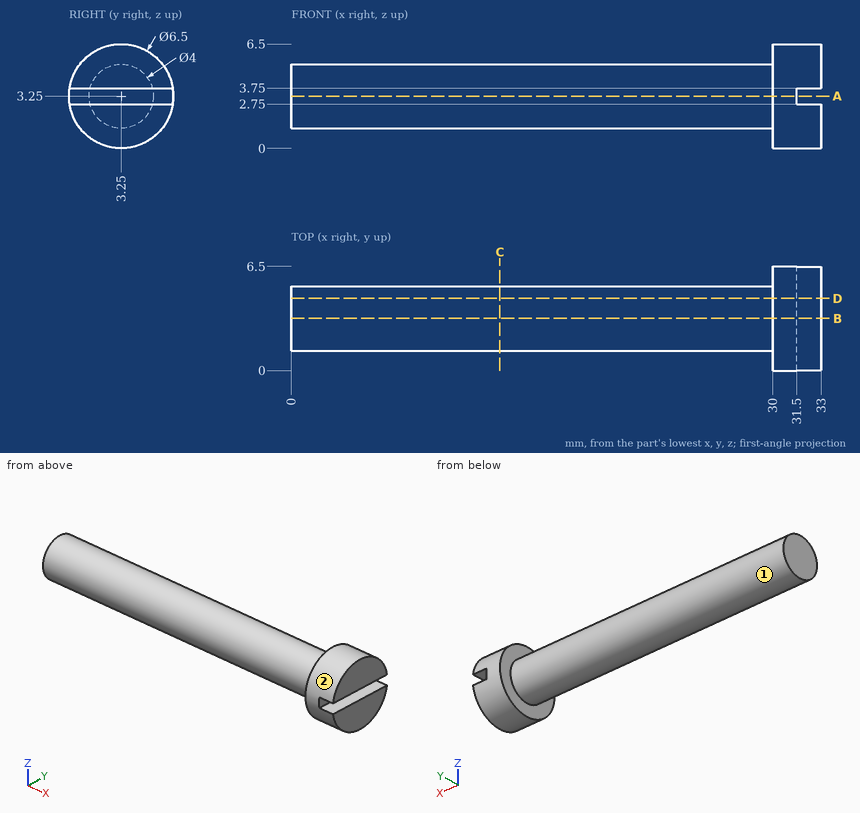
Source: three-view drawing plus pictorial views. Frame: mm from the lowest corner of the part. A direction names the side the tool comes from. Give positions to 0.01 mm unless a question says otherwise; leave off trailing zeros. Write each loop counter-clockwise with the first axis right and the second up, starting at its lowest first coordinate (ties: lowest second). Pieces come first, ordered by that corner, then holes. Notation, with made-up numbers: (35, 27) -> (81, 27) arc R34 cw to (81, 61) -> close; hole circle Ø1 at (18.25, 41.5). An arc over 180 degrees is marked (long way). Answer in a Markdown table with one row per item.
(1) Ray query, line 1 along X through (y, z) = (5.5, 3); line 2 along Z through (x, y) = (3, 1.5); line 3 along Y through (x, z) = (2.5, 3). Return the intervals inside material, ascending. Write a range as [from, to].
Answers below:
| item | result |
|---|---|
| line 1 | [30, 31.5] |
| line 2 | [2.28, 4.22] |
| line 3 | [1.27, 5.23] |
(2) Set-up query: the marked faces 1 and 2. Return all of +Z, -Z, +X, -X, +Y, -Y with unobstructed straight access to the full face (end or side cutting, diameter ignored); none if empty.
Answers below:
| item | result |
|---|---|
| face 1 | -X |
| face 2 | +X, -X |
(3) Section query D-D on y = 4.5. Return loops of the section in (x, z), then the cut area to 3 significant figures.
Answers below:
| item | result |
|---|---|
| outline | (0, 1.69) -> (30, 1.69) -> (30, 0.25) -> (33, 0.25) -> (33, 2.75) -> (31.5, 2.75) -> (31.5, 3.75) -> (33, 3.75) -> (33, 6.25) -> (30, 6.25) -> (30, 4.81) -> (0, 4.81) -> close |
| area | 110 mm^2 |
(4) Section query B-B on y = 3.25. Return loops of the section in (x, z).
Answers below:
| item | result |
|---|---|
| outline | (0, 1.25) -> (30, 1.25) -> (30, 0) -> (33, 0) -> (33, 2.75) -> (31.5, 2.75) -> (31.5, 3.75) -> (33, 3.75) -> (33, 6.5) -> (30, 6.5) -> (30, 5.25) -> (0, 5.25) -> close |
(5) Section query C-C on x = 13. Return loops of the section in (y, z).
Answers below:
| item | result |
|---|---|
| outline | circle Ø4 at (3.25, 3.25) |
(6) Section query A-A on z = 3.25. Return loops of the section in (x, y), then the cut area to 3 significant figures.
Answers below:
| item | result |
|---|---|
| outline | (0, 1.25) -> (30, 1.25) -> (30, 0) -> (31.5, 0) -> (31.5, 6.5) -> (30, 6.5) -> (30, 5.25) -> (0, 5.25) -> close |
| area | 130 mm^2 |
(7) Pin query (flat end, axial travel): pin 1 (0.8 mm diameter, centred on x = 32.5, y = 2.5, fed in from -Z); pin 2 (3 mm diameter, centred on x = 27.5, y = 2, fed in from +Z); pin 3 (1 mm diameter, centred on x = 26.5, y = 5.5, fed in from +Z). Return the tip coordinate at first contact, or that it passes through.
Answers below:
| item | result |
|---|---|
| pin 1 | z = 0.02 |
| pin 2 | z = 5.25 |
| pin 3 | z = 4.22 |
